Part model, mm, in its own coordinate system. A direction names the side the tool comes from. Give positions to 0.01 mm unless a question says otherwise; leave off trailing zeros. Order: outer loops, then holes, each group sorted by start corner. A loop starts at its lowest first (then second) coordinate and runs counter-clockwise, first axis right, second up.
1. Slice it at C-C on y = -1.45. List the corners of the cut face in (x, z) (1 decimal), and give its area (3 significant figures).
2. Probe line 1 (X direction, y = -2.25, z = 6.75); line 2 (Z direction, x = 20.5, y = -2.25) (3 decimals). List the from-to ranges inside material, lowest first.
3. Slice it at A-A on x = 16. List the corners of the cut face in (y, z) (3 decimals), and give its area (3 significant figures).
4. Which spindle directions (+Z, -Z, +X, -X, +Y, -Y) get a long thin tool onto all of the face, cutting with end or side? Do faces 1 (the flat face through (16, -1, 0)), 2 (the flat face through (4.33, -1, 9)). Say none if no direction does.
5. Mould opens along X. For faces 3 (the flat face through (16, -1, 18.11)), 4 (the flat face through (28.87, -1, 9)), 5 (the flat face through (0, -1, 9)) say: +X half, -X half, draft (parallel to the pull), parting line (faces both ways), or undercut.
6. Slice it at B-B on z = 8.75. List the corners of the cut face in (x, y), and give its area (3 significant figures).
7. Drop a flat-ended pin along its axis: pin 1 Ø0.8 at (x, y) = (21.5, -1) entering from -Z. Give the stop position or say it passes through.
from build123d import *

# Parameters (mm, degrees)
SKETCH_W        = 33.2
SKETCH_H        = 18.11
PAD_DEPTH       = 2.6
SKETCH002_W     = 24.54
SKETCH002_H     = 12.56
POCKET_DEPTH    = 2.6
SKETCH003_R     = 0.5
POCKET001_DEPTH = 5


with BuildPart() as part:
    # Sketch → Pad (new body)
    with BuildSketch(Plane.XZ):
        with Locations((16.6, 9.055)):
            Rectangle(SKETCH_W, SKETCH_H)
    extrude(amount=PAD_DEPTH)

    # Sketch002 (on Face6 of Pad) → Pocket (cut)
    with BuildSketch(Plane.XZ.offset(2.6)):
        with Locations((16.6, 9.055)):
            Rectangle(SKETCH002_W, SKETCH002_H)
    extrude(amount=-POCKET_DEPTH, mode=Mode.SUBTRACT)

    # Sketch003 (on Face4 of Pocket) → Pocket001 (cut)
    with BuildSketch(Plane(origin=(0, 0, 0), x_dir=(1, 0, 0), z_dir=(0, 1, 0))):
        with Locations((31.0215, -16.715)):
            Circle(SKETCH003_R)
    extrude(amount=-POCKET001_DEPTH, mode=Mode.SUBTRACT)


solid = part.part
Data:
1. outline: (0, 0) - (33.2, 0) - (33.2, 18.1) - (0, 18.1) - close; hole (4.3, 2.8) - (28.9, 2.8) - (28.9, 15.3) - (4.3, 15.3) - close; hole circle Ø1 at (31, 16.7)
1. area: 292 mm2
2. line 1: x = 0 to 4.33, 28.87 to 33.2
2. line 2: z = 0 to 2.775, 15.335 to 18.11
3. outline: (-2.6, 0) - (0, 0) - (0, 2.775) - (-2.6, 2.775) - close; (-2.6, 15.335) - (0, 15.335) - (0, 18.11) - (-2.6, 18.11) - close
3. area: 14.4 mm2
4. face 1: -Z, +X, -X, +Y, -Y
4. face 2: +Y, -Y
5. face 3: draft
5. face 4: undercut
5. face 5: -X half
6. outline: (0, -2.6) - (4.33, -2.6) - (4.33, 0) - (0, 0) - close; (28.87, -2.6) - (33.2, -2.6) - (33.2, 0) - (28.87, 0) - close
6. area: 22.5 mm2
7. pin 1: stops at z = 0
